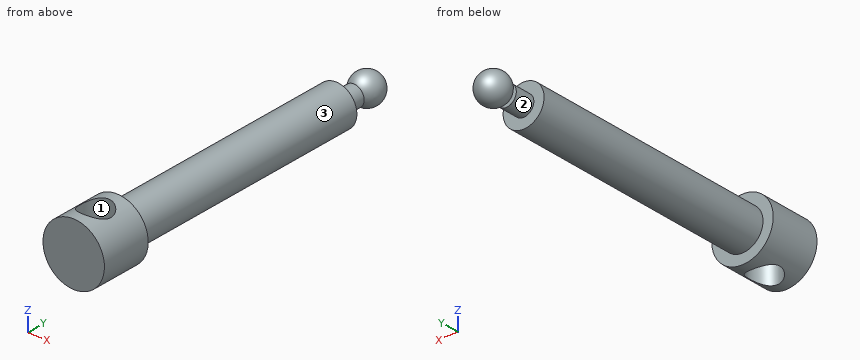
```python
from build123d import *

# Parameters (mm, degrees)
SZKIC1_R                        = 2
DODANIE_WYCI_GNI_CIE1_DEPTH     = 25
SZKIC2_R                        = 1
DODANIE_WYCI_GNI_CIE2_DEPTH     = 2
SZKIC4_R                        = 3
DODANIE_WYCI_GNI_CIE3_DEPTH     = 5
WYTNIJ_WYCI_GNI_CIE1_DEPTH      = 31.272564199
WYTNIJ_WYCI_GNI_CIE1_DEPTH_BACK = 31.272564199
SZKIC5_R                        = 1.5


with BuildPart() as part:
    # Szkic1 → Dodanie-wyciągnięcie1 (new body)
    with BuildSketch(Plane(origin=(0, 0, 0), x_dir=(1, 0, 0), z_dir=(0, 1, 0))):
        with Locations(Location((0, 0, 0), (0, 0, 270))):
            Circle(SZKIC1_R)
    extrude(amount=DODANIE_WYCI_GNI_CIE1_DEPTH)

    # Szkic2 → Dodanie-wyciągnięcie2 (add)
    with BuildSketch(Plane(origin=(0, 25, 0), x_dir=(1, 0, 0), z_dir=(0, 1, 0))):
        with Locations(Location((0, 0, 0), (0, 0, 270))):
            Circle(SZKIC2_R)
    extrude(amount=DODANIE_WYCI_GNI_CIE2_DEPTH)

    # Szkic3 → Obrót3 (revolve)
    with BuildSketch(Plane.XY):
        with BuildLine():
            Line((0, 29.973790938), (0, 26.973790938))
            ThreePointArc((0, 26.973790938), (1.5, 28.473790938), (0, 29.973790938))
        make_face()
    revolve(axis=Axis((0, 0, 0), (0, 1, 0)))

    # Szkic4 → Dodanie-wyciągnięcie3 (add)
    with BuildSketch(Plane.XZ):
        with Locations(Location((0, 0, 0), (0, 0, 270))):
            Circle(SZKIC4_R)
    extrude(amount=DODANIE_WYCI_GNI_CIE3_DEPTH)

    # Szkic5 → Wytnij-wyciągnięcie1 (cut, two sides: drawn at the far end of the back side and taken through both)
    with BuildSketch(Plane.XY.offset(-WYTNIJ_WYCI_GNI_CIE1_DEPTH_BACK)):
        with Locations(Location((0, -2.5, 0), (0, 0, 270.000000001))):
            Circle(SZKIC5_R)
    extrude(amount=WYTNIJ_WYCI_GNI_CIE1_DEPTH + WYTNIJ_WYCI_GNI_CIE1_DEPTH_BACK, mode=Mode.SUBTRACT)


solid = part.part
```
Source: CAD feature listing. Evaluate the final solid. Frame: model axes, mm. Face numbers are marked on the shaded views. A direction names the side the tool comes from. Give positions to 0.01 mm unless a question says otherwise; leave off trailing zeros. Order: outer loops, then holes, each group sorted by start corner. A loop starts at its lowest first (then second) coordinate and runs counter-clockwise, first axis right, second up. Notation, with made-up numbers: (87.5, 17.25) -> (91.5, 17.25) arc R28 cw to (91.5, 39.25) -> close; hole circle Ø6 at (1.5, -5). An arc over 180 degrees is marked (long way). Use a Markdown table: item, result.
Q1. Access query for the marked faces 1, 2 and 3. Directions: +Z, -Z, +X, -X, +Y, -Y. A direction counts if a zero-diameter tool reaches every point of the face in a straight line with its end or side. Return the directions, or none.
A:
| item | result |
|---|---|
| face 1 | +Z, -Z |
| face 2 | none |
| face 3 | +Y |
Q2. Material intervals for line 1 (Y direction, x = 0.25, z = -1); line 2 (X direction, y = -2.5, z = 0); line 3 (Y direction, x = -1, z = 2), sorted ascending. Write a range as [from, to].
A:
| item | result |
|---|---|
| line 1 | [-5, -3.98], [-1.02, 25], [27.38, 29.56] |
| line 2 | [-3, -1.5], [1.5, 3] |
| line 3 | [-5, -3.62], [-1.38, 0] |
Q3. First-contact query: P1, Ø1, axis at x = 2, y = 16.5, coming from the +Z side; P2, Ø1.5, axis at x = 2, y = 11, coming from the +Z side; P3, Ø3, axis at x = 1, y = 2.5, coming from the +Z side; P4, Ø1, axis at x = 2.5, z = 2.5, coming from the +Y side. Flat tips, straight axial feed; report the tip coordinate or a pass-through.
A:
| item | result |
|---|---|
| P1 | z = 1.32 |
| P2 | z = 1.56 |
| P3 | z = 2 |
| P4 | through |
Q4. Section B-B (y = -2.5). Return the cut outline in (x, z), and give its area (3 significant figures).
A:
| item | result |
|---|---|
| outline | (-1.5, -2.6) -> (-1.5, 2.6) arc R3 ccw to start; (1.5, -2.6) arc R3 ccw to (1.5, 2.6) -> close |
| area | 11.1 mm^2 |
Q5. Section C-C (y = 6.5). Return the cut outline in (x, z), and give its area (3 significant figures).
A:
| item | result |
|---|---|
| outline | circle Ø4 at (0, 0) |
| area | 12.6 mm^2 |
Q6. Section A-A (z = -2.5). Return the cut outline in (x, y).
A:
| item | result |
|---|---|
| outline | (-1.66, -5) -> (1.66, -5) -> (1.66, 0) -> (-1.66, 0) -> close; hole circle Ø3 at (0, -2.5) |
Q7. Section D-D (z = 0). Return the cut outline in (x, y), and give its area (3 significant figures).
A:
| item | result |
|---|---|
| outline | (-3, -5) -> (3, -5) -> (3, 0) -> (2, 0) -> (2, 25) -> (1, 25) -> (1, 27) -> (0.28, 27) arc R1.5 ccw (long way) to (-0.28, 27) -> (-1, 27) -> (-1, 25) -> (-2, 25) -> (-2, 0) -> (-3, 0) -> close; hole circle Ø3 at (0, -2.5) |
| area | 134 mm^2 |
